from build123d import *

# Parameters (mm, degrees)
SKETCH1_R                = 4
BOSS_EXTRUDE1_DEPTH      = 37
BOSS_EXTRUDE1_DEPTH_BACK = 37
CUT_EXTRUDE1_DEPTH       = 30


with BuildPart() as part:
    # Sketch1 → Boss-Extrude1 (new body, two sides)
    with BuildSketch(Plane(origin=(0, 0, 0), x_dir=(1, 0, 0), z_dir=(0, 1, 0))) as boss_extrude1_sk:
        Circle(SKETCH1_R)
    extrude(amount=BOSS_EXTRUDE1_DEPTH)
    extrude(boss_extrude1_sk.sketch, amount=-BOSS_EXTRUDE1_DEPTH_BACK)

    # Sketch2 → Cut-Extrude1 (cut)
    with BuildSketch(Plane(origin=(0, 37, 0), x_dir=(1, 0, 0), z_dir=(0, 1, 0))):
        Polygon((-32.617462983, 2), (-3.464101615, 2), (3.464101615, 2), (32.617462983, 2), (32.617462983, 60.306722736), (-32.617462983, 60.306722736), align=None)
    cut_extrude1 = extrude(amount=-CUT_EXTRUDE1_DEPTH, mode=Mode.SUBTRACT)

    # Mirror1: Cut-Extrude1 across plane
    add(cut_extrude1.mirror(Plane.ZX), mode=Mode.SUBTRACT)


solid = part.part
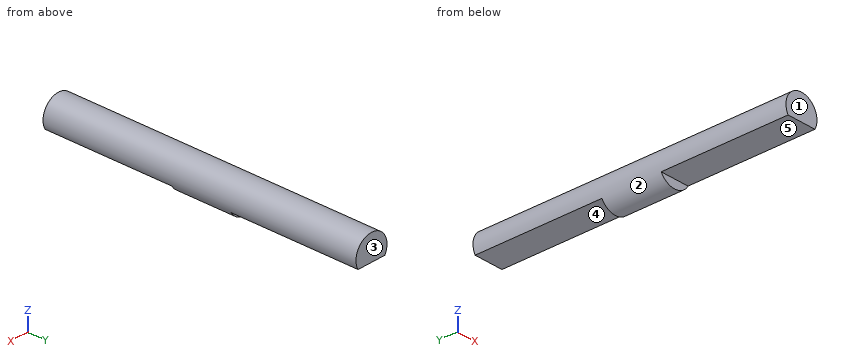
Geometry check sheet. Reference: the model listing, model coordinates, mm. Face numbers are marked on the shaded views. A direction names the side the tool comes from. Give positions to 0.01 mm unless a question says otherwise; leave off trailing zeros. Loops run counter-clockwise (first coordinate to the right, second up) from the corner with the lowest first, then second, coordinate; pieces in that order, holes last.
(1) Release check for a two-part mould opening along X. For the marked faces 1 and 2 record: released by +X, released by -X, zero draft, split by the parting line, or undercut.
From the geometry:
face 1: zero draft
face 2: split by the parting line
(2) Set-up check for the marked faces 3, 4 and 5: record each of +Z, -Z, +X, -X, +Y, -Y from which the full face is reachable in a straight line by a thin tool's end or side.
From the geometry:
face 3: +Z, -Z, +X, -X, +Y
face 4: -Z, +X, -X, +Y
face 5: -Z, +X, -X, -Y
(3) Section check B-B on y = -21. Record the cut outline in (x, z), then the cut area to 3 significant figures.
From the geometry:
outline: (-3.46, -2) - (3.46, -2) arc R4 ccw (long way) to start
area: 40.4 mm2
(4) Depth check by flat-ended pin: pin 1 Ø1 at (y, z) = (-14.5, -0.5) entering from -X; pin 2 Ø3.5 at (x, y) = (1.5, -16) entering from -Z; pin 3 Ø1 at (x, z) = (0, -3.5) entering from -Y; pin 4 Ø3 at (x, y) = (-2.5, 22.5) entering from +Z. Enter the tip coordinate at first touch or a pass-through.
From the geometry:
pin 1: stops at x = -4
pin 2: stops at z = -2
pin 3: stops at y = -7
pin 4: stops at z = 3.87
(5) Section check D-D on x = 2.75. Record the cut outline in (y, z).
From the geometry:
outline: (-37, -2) - (-7, -2) - (-7, -2.9) - (7, -2.9) - (7, -2) - (37, -2) - (37, 2.9) - (-37, 2.9) - close
(6) Section check C-C on z = 2.5. Record the cut outline in (x, y), then the cut area to 3 significant figures.
From the geometry:
outline: (-3.12, -37) - (3.12, -37) - (3.12, 37) - (-3.12, 37) - close
area: 462 mm2
(7) Thickness scan on L1, parallel to Y at x = -1.75, z = -2.5; L2, parallel to Z at x = -0.25, y = 5.5; L3, parallel to Z at x = -2, y = -30.5. Record the ranges inside material, lowest first.
From the geometry:
L1: y = -7 to 7
L2: z = -3.99 to 3.99
L3: z = -2 to 3.46
(8) Section check A-A on x = 0. Record the cut outline in (y, z), then the cut area to 3 significant figures.
From the geometry:
outline: (-37, -2) - (-7, -2) - (-7, -4) - (7, -4) - (7, -2) - (37, -2) - (37, 4) - (-37, 4) - close
area: 472 mm2
